Geometry check sheet. Reference: the model listing, model coordinates, mm. A direction names the side the tool comes from. Give positions to 0.01 mm unless a question says otherwise; leave off trailing zeros. Loops run counter-clockwise (first coordinate to the right, second up) from the corner with the lowest first, then second, coordinate; pieces in that order, holes last. Notation, with made-up numbers: (31, 74) -> (59, 74) arc R8 cw to (59, 86) -> close; hole circle Ø5 at (-9.5, 46). An arc over 180 degrees is marked (long way). Write each question's results on one line, items separated by ' | '. Start each with the question number.
1) Sectioned sample at B-B on z = 11. Record the cut outline in (x, y) (1 decimal), then the cut area to 3 significant figures.
2) Draft check along Y on faces 6 (the face through (3.16, 87.32, 8.77)), 7 (the face through (2, 0, 0)), 8 (the face through (11.713, 66.089, 11.519)), 9 (the face through (2.164, 1.533, 24.934)). Enter one of: pulls with the +Y half, pulls with the -Y half, needs draft (parallel to the pull), parting line crosses it, or undercut.
3) Depth check by flat-ended pin: pin 1 (8.5 mm diameter, centred on y = -11.5, z = 34.5, fed in from -X); pin 2 (20.5 mm diameter, centred on x = 0, y = 67.5, fed in from +Z); pin 3 (10.5 mm diameter, centred on x = 2, z = 44.5, fed in from +Y); pin 4 (5.5 mm diameter, centred on x = 2.31, z = 45.34, fed in from +Y) (1 decimal). Enter the tip coordinate at first touch or a pass-through.
4) Set-up check for faces 1 (the face through (2, 36.744, 37)), 2 (the face through (3, 63, 5.08)), 3 (the face through (2, -36.242, 37)), 4 (the face through (12.812, 0, 22)), 5 (the face through (2, -9.076, 40)): record each of +Z, -Z, +X, -X, +Y, -Y from which the full face is reachable in a straight line by a thin tool's end or side.
5) Sectioned sample at C-C on y = 66. Record the cut outline in (x, z), then the cut area to 3 significant figures.
6) Sectioned sample at D-D on y = -25.5. Record the cut outline in (x, z), then the cut area to 3 significant figures.
7) Sectioned sample at A-A on x = 0. Record the cut outline in (y, z).
8) Scan lines: line 1 (Z direction, x = 2, y = 24); line 2 (Y direction, x = 8.5, z = 5.5); line 3 (Y direction, x = -4, z = 44.5). Record each from-to range of solid material in increasing order. Write a range as from..to.
```python
from build123d import *

# Parameters (mm, degrees)
F1_DEPTH  = 17.78
F2_R      = 8.961227
F2_R_2    = 9.35653
F3_DEPTH  = 12.7
F4_W      = 21.001198
F4_H      = 72.985793
F5_DEPTH  = 38.1
F7_DEPTH  = 126.068455
F9_DEPTH  = 32.372704
F10_R     = 4.654821
F11_DEPTH = 126.068455


with BuildPart() as f1:
    # F0 (on Top) → F1 (new body)
    with BuildSketch(Plane.XY):
        with BuildLine():
            ThreePointArc((-18.604314, -75.995304), (2.788962, -89.323594), (24.182238, -75.995304))
            Line((24.182238, -75.995304), (24.182238, 74.255139))
            ThreePointArc((24.182238, 74.255139), (2.788962, 87.323361), (-18.604314, 74.255139))
            Line((-18.604314, 74.255139), (-18.604314, -75.995304))
        make_face()
    extrude(amount=F1_DEPTH)

    # F2 (on face) → F3 (cut)
    with BuildSketch(Plane.XY.offset(17.78)):
        with Locations((2.788962, -65.490246)):
            Circle(F2_R)
        with Locations((2.788962, 63.278366)):
            Circle(F2_R_2)
    extrude(amount=-F3_DEPTH, mode=Mode.SUBTRACT)

    # F4 (on face) → F5 (join)
    with BuildSketch(Plane.XY.offset(17.78)):
        with Locations((2.311133, 0.250964)):
            Rectangle(F4_W, F4_H)
    extrude(amount=F5_DEPTH)

    # F6 (on face) → F7 (cut, through all)
    with BuildSketch(Plane(origin=(0, 36.743861, 0), x_dir=(-1, 0, 0), z_dir=(0, 1, 0))):
        with BuildLine():
            Line((8.189466, 55.88), (-2.311133, 55.88))
            ThreePointArc((-2.311133, 55.88), (4.823938, 53.096615), (8.189466, 46.216957))
            Line((8.189466, 46.216957), (8.189466, 55.88))
        make_face()
        with BuildLine():
            Line((-12.811732, 55.88), (-12.811732, 46.216957))
            ThreePointArc((-12.811732, 46.216957), (-9.446204, 53.096615), (-2.311133, 55.88))
            Line((-2.311133, 55.88), (-12.811732, 55.88))
        make_face()
    extrude(amount=-F7_DEPTH, mode=Mode.SUBTRACT)

    # F8 (on face) → F9 (cut, through all)
    with BuildSketch(Plane(origin=(-8.189466, 0, 0), x_dir=(0, -1, 0), z_dir=(-1, 0, 0))):
        with BuildLine():
            Line((9.075661, 56.156088), (-11.796514, 56.156088))
            Line((-11.796514, 56.156088), (-11.796514, 30.562826))
            ThreePointArc((-11.796514, 30.562826), (-1.360426, 24.932368), (9.075661, 30.562826))
            Line((9.075661, 30.562826), (9.075661, 56.156088))
        make_face()
    extrude(amount=-F9_DEPTH, mode=Mode.SUBTRACT)

    # F10 (on face) → F11 (cut, through all)
    with BuildSketch(Plane(origin=(0, 36.743861, 0), x_dir=(-1, 0, 0), z_dir=(0, 1, 0))):
        with Locations((-2.311133, 45.343103)):
            Circle(F10_R)
    extrude(amount=-F11_DEPTH, mode=Mode.SUBTRACT)


solid = f1.part
```
Result:
1) outline: (-18.6, -76) arc R23.8 ccw to (24.2, -76) -> (24.2, 74.3) arc R24 ccw to (-18.6, 74.3) -> close; hole circle Ø18.7 at (2.8, 63.3); hole circle Ø17.9 at (2.8, -65.5) | area: 6,710 mm^2
2) face 6: pulls with the +Y half | face 7: needs draft | face 8: undercut | face 9: undercut
3) pin 1: x = -8.19 | pin 2: z = 17.78 | pin 3: y = 36.74 | pin 4: through
4) face 1: +Z, +X, -X, +Y | face 2: +Z | face 3: +Z, +X, -X, -Y | face 4: +Z, +X, +Y, -Y | face 5: +Z, +X, -X
5) outline: (-18.6, 0) -> (24.18, 0) -> (24.18, 17.78) -> (11.74, 17.78) -> (11.74, 5.08) -> (-6.16, 5.08) -> (-6.16, 17.78) -> (-18.6, 17.78) -> close | area: 533 mm^2
6) outline: (-18.6, 0) -> (24.18, 0) -> (24.18, 17.78) -> (12.81, 17.78) -> (12.81, 46.22) arc R10.54 ccw to (2.31, 55.88) arc R10.54 ccw to (-8.19, 46.22) -> (-8.19, 17.78) -> (-18.6, 17.78) -> close; hole circle Ø9.31 at (2.31, 45.34) | area: 1,450 mm^2
7) outline: (-89.16, 0) -> (87.16, 0) -> (87.16, 17.78) -> (72.21, 17.78) -> (72.21, 5.08) -> (54.35, 5.08) -> (54.35, 17.78) -> (36.74, 17.78) -> (36.74, 41.3) -> (11.8, 41.3) -> (11.8, 30.56) arc R12.49 cw to (-9.08, 30.56) -> (-9.08, 41.3) -> (-36.24, 41.3) -> (-36.24, 17.78) -> (-56.97, 17.78) -> (-56.97, 5.08) -> (-74.01, 5.08) -> (-74.01, 17.78) -> (-89.16, 17.78) -> close; (-36.24, 49.38) -> (-9.08, 49.38) -> (-9.08, 55.62) -> (-36.24, 55.62) -> close; (11.8, 49.38) -> (36.74, 49.38) -> (36.74, 55.62) -> (11.8, 55.62) -> close
8) line 1: 0..40.7, 49.99..55.88 | line 2: -88.63..-72.4, -58.58..55.87, 70.69..86.64 | line 3: -36.24..-9.08, 11.8..36.74
